Build history of the part. All positions in model axes, mm. A direction names the side the tool comes from. Coordinates: 2 decimals unless noted, no trailing zeros. Loops run counter-clockwise (first coordinate to the right, second up) from the corner with the lowest first, then second, coordinate; pieces in that order, holes last.
(1) Tool access for faces 4 (the face through (26, 0, 57.15)), 5 (the face through (12.65, -3.864, -60.281)): list every direction of +Z, -Z, +X, -X, +Y, -Y with a clear straight run to the whole face (end or side of a thin tool).
(2) Flat gauge pin, fed straight in: P1, Ø16, axis at y = 6.5, z = 8.5, coming from the +X side (3 decimals). Where does the tip first touch, or does it go through?
(3) Slice it at B-B (y = 0). Give the cut face in (x, z) (3 decimals), and give its area (3 significant figures).
(4) Two-plate mould, pull along Z, no slides. Class faces 1 (the face through (12, -4, 63.5)), 2 (the face through (26, 0, -57.15)), 3 (the face through (34.925, 0, 60)): pulls with the +Z half, pulls with the -Z half, needs draft (parallel to the pull), parting line crosses it, or undercut.
(5) Wall check: L1, parallel to Z at x = 11, y = -5.5; L2, parallel to X at y = 11.5, z = 6 (3 decimals). Give the ranges that are in metal, low to high.
(6) Slice it at C-C (y = -14). Give the cut face in (x, z) (3 decimals).
(7) Slice it at D-D (x = 15). Give the cut face in (y, z) (3 decimals).
(8) Slice it at A-A (x = 32.5). Give the cut face in (y, z) (3 decimals).
from build123d import *

# Parameters (mm, degrees)
F0_W     = 31.75
F0_H     = 6.35
F1_DEPTH = 15.875
F2_R     = 6.35
F3_DEPTH = 127


with BuildPart() as f1:
    # F0 (on Front) → F1 (new body, symmetric)
    with BuildSketch(Plane.XZ):
        with Locations((19.05, -60.325)):
            Rectangle(F0_W, F0_H)
        Polygon((3.175, 63.5), (-3.175, 63.5), (-3.175, -63.5), (3.175, -63.5), (3.175, -57.15), (3.175, 57.15), align=None)
        with Locations((19.05, 60.325)):
            Rectangle(F0_W, F0_H)
    extrude(amount=F1_DEPTH, both=True)

    # F2 (on Top) → F3 (cut, symmetric)
    with BuildSketch(Plane.XY):
        with Locations((17.689286, 0)):
            Circle(F2_R)
    extrude(amount=F3_DEPTH, both=True, mode=Mode.SUBTRACT)


solid = f1.part
Response values:
1. face 4: +X, +Y, -Y
1. face 5: +Z, -Z
2. P1: stops at x = 3.175
3. outline: (-3.175, -63.5) - (11.339, -63.5) - (11.339, -57.15) - (3.175, -57.15) - (3.175, 57.15) - (11.339, 57.15) - (11.339, 63.5) - (-3.175, 63.5) - close; (24.039, -63.5) - (34.925, -63.5) - (34.925, -57.15) - (24.039, -57.15) - close; (24.039, 57.15) - (34.925, 57.15) - (34.925, 63.5) - (24.039, 63.5) - close
3. area: 1,050 mm2
4. face 1: pulls with the +Z half
4. face 2: undercut
4. face 3: needs draft
5. L1: z = -63.5 to -57.15, 57.15 to 63.5
5. L2: x = -3.175 to 3.175
6. outline: (-3.175, -63.5) - (34.925, -63.5) - (34.925, -57.15) - (3.175, -57.15) - (3.175, 57.15) - (34.925, 57.15) - (34.925, 63.5) - (-3.175, 63.5) - close
7. outline: (-15.875, -63.5) - (-5.752, -63.5) - (-5.752, -57.15) - (-15.875, -57.15) - close; (-15.875, 57.15) - (-5.752, 57.15) - (-5.752, 63.5) - (-15.875, 63.5) - close; (5.752, -63.5) - (15.875, -63.5) - (15.875, -57.15) - (5.752, -57.15) - close; (5.752, 57.15) - (15.875, 57.15) - (15.875, 63.5) - (5.752, 63.5) - close
8. outline: (-15.875, -63.5) - (15.875, -63.5) - (15.875, -57.15) - (-15.875, -57.15) - close; (-15.875, 57.15) - (15.875, 57.15) - (15.875, 63.5) - (-15.875, 63.5) - close
